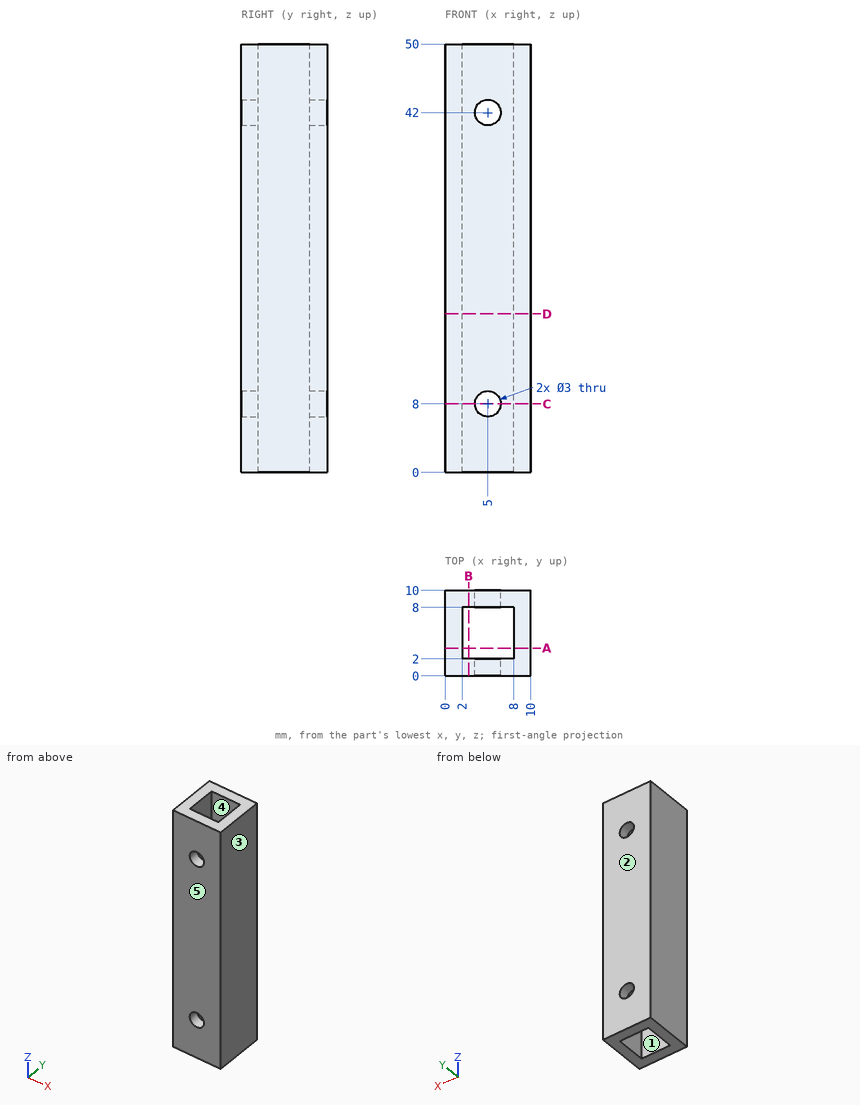
Source: three-view drawing plus pictorial views. Frame: mm from the lowest corner of the part. A direction names the side the tool comes from. Coordinates: 2 decimals unless noted, no trailing zeros. Loops run counter-clockwise (first coordinate to the right, second up) from the corner with the lowest first, then second, coordinate; pieces in that order, holes last. Notation, with made-up numbers: (12.25, 26.25) -> (35.25, 26.25) arc R9 cw to (35.25, 39.25) -> close; hole circle Ø2 at (64, 28). An arc over 180 degrees is marked (long way). One line per item, written item: value.
(1) Cut plane D-D (z = 18.5). Output: boundary loops of the cut face in (x, y).
Answer below:
outline: (0, 0) -> (10, 0) -> (10, 10) -> (0, 10) -> close; hole (2, 2) -> (8, 2) -> (8, 8) -> (2, 8) -> close
(2) Ray query, line 1 along X through (y, z) = (3, 30.5); line 2 along X through (y, z) = (9.4, 42). Return the intervals inside material, ascending.
Answer below:
line 1: x = 0 to 2, 8 to 10
line 2: x = 0 to 3.5, 6.5 to 10
(3) Set-up query: the marked faces 4 and 5. Return all of +Z, -Z, +X, -X, +Y, -Y with unobstructed straight access to the full face (end or side cutting, diameter ignored); none if empty.
Answer below:
face 4: +Z, -Z
face 5: +Z, -Z, +X, -X, -Y
(4) Cut plane C-C (z = 8). Output: boundary loops of the cut face in (x, y), then the cut area to 3 significant figures.
Answer below:
outline: (0, 0) -> (3.5, 0) -> (3.5, 2) -> (2, 2) -> (2, 8) -> (3.5, 8) -> (3.5, 10) -> (0, 10) -> close; (6.5, 0) -> (10, 0) -> (10, 10) -> (6.5, 10) -> (6.5, 8) -> (8, 8) -> (8, 2) -> (6.5, 2) -> close
area: 52.0 mm2
(5) Cut plane A-A (y = 3.25). Output: boundary loops of the cut face in (x, z), then the cut area to 3 significant figures.
Answer below:
outline: (0, 0) -> (2, 0) -> (2, 50) -> (0, 50) -> close; (8, 0) -> (10, 0) -> (10, 50) -> (8, 50) -> close
area: 200 mm2
(6) Draft query along Y for the marked faces 1, 2 and 3. Return one class per face: pulls with the +Y half, pulls with the -Y half, needs draft (parallel to the pull), parting line crosses it, or undercut.
Answer below:
face 1: undercut
face 2: pulls with the +Y half
face 3: needs draft
